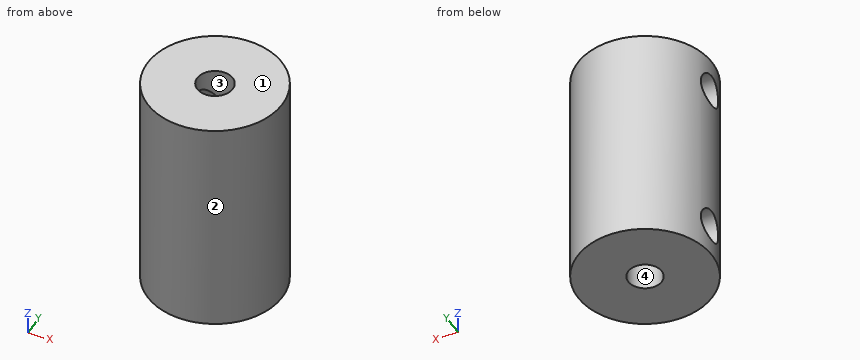
Autodesk Inventor part; units mm, degrees
ref_plane "YZ Plane" through (0, 0, 0) normal (1, 0, 0) x (0, 1, 0)
ref_plane "XZ Plane" through (0, 0, 0) normal (0, 1, 0) x (-1, 0, 0)
ref_plane "XY Plane" through (0, 0, 0) normal (0, 0, 1) x (1, 0, 0)
sketch "Sketch1" plane through (0, 0, 0) normal (0, 0, 1) x (1, 0, 0)
  circle A0 centre (0, 0) radius 6
  dimension "d0" = 12
extrude "Extrusion1" add sketch "Sketch1" along normal blind 20
sketch "Sketch2" plane through (0, 0, 20) normal (0, 0, 1) x (1, 0, 0)
  circle A0 centre (0, 0) radius 1.585
  dimension "d3" = 3.17
extrude "Extrusion2" cut sketch "Sketch2" against normal blind 10
sketch "Sketch3" plane through (0, 0, 0) normal (0, 0, -1) x (-1, 0, 0)
  circle A0 centre (0, 0) radius 1.5
  dimension "d6" = 3
extrude "Extrusion3" cut sketch "Sketch3" against normal blind 10
sketch "Sketch4" plane through (0, 0, 0) normal (1, 0, 0) x (0, 1, 0)
  circle A0 centre (0, 17) radius 1.5
  circle A1 centre (0, 3) radius 1.5
  line L0 (6, 20) -> (-6, 20)
  point P0 (0, 0)
  dimension "d9" = 3
  dimension "d10" = 3
  dimension "d11" = 3
extrude "Extrusion4" cut sketch "Sketch4" against normal through all
equation "\"d11\" = d10"
properties part number "3mm_.125inch_ShaftCoupler" material "Aluminum 6061"
Geometry check sheet. Reference: the model listing, model coordinates, mm. Face numbers are marked on the shaded views. Coordinates: 2 decimals unless noted, no trailing zeros. Write each loop counter-clockwise with the first axis right and the second up, starting at its lowest first coordinate (ties: lowest second). Pieces come first, ordered by that corner, then holes. Notation, with made-up numbers: M -29,74.5 L -25,74.5 A22 cw -25,97.5 Z; hole C -31.75,9 d6. An arc over 180 degrees is marked long. Use one line per item in the form item = value. Start each with the question number.
1) Go/stop test with a flat-tipped pin: pin 1 Ø3.5 at (x, y) = (0, 0) entering from -Z. Record where the tip stops, or that it passes through.
2) Release check for a two-part mould opening along Y. For the marked faces 1, 2, 3 and 4 record: pulls with the +Y half, pulls with the -Y half, needs draft (parallel to the pull), parting line crosses it, or undercut.
3) Section check D-D on z = 17. Enter the section's corners in (x, y) (3 decimals), and give its area (3 significant figures).
4) Section check A-A on y = 0. Enter the section's corners in (x, z) (3 decimals), and give its area (3 significant figures).
5) Thickness scan on probe 1 along X at (y, z) = (0, 12.75) (3 decimals); probe 2 along Y at (x, z) = (0, 3.5); probe 3 along X at (y, z) = (0, 16.75) (3 decimals). Record the ranges inside material, lowest first. Write a range as from..to.
6) Section check C-C on z = 5.5. Enter the section's corners in (x, y), and give its area (3 significant figures).
7) Section check B-B on x = -3.25. Enter the section's corners in (y, z).
Responses:
q1.pin_1 = 0
q2.face_1 = needs draft
q2.face_2 = parting line crosses it
q2.face_3 = undercut
q2.face_4 = undercut
q3.outline = M -5.809,-1.5 A6 ccw long -5.809,1.5 L -0.512,1.5 A1.585 cw long -0.512,-1.5 Z
q3.area = 91.3 mm2
q4.outline = M -6,0 L -1.5,0 L -1.5,1.5 L -6,1.5 Z; M -6,4.5 L -1.5,4.5 L -1.5,10 L -1.585,10 L -1.585,15.5 L -6,15.5 Z; M -6,18.5 L -1.585,18.5 L -1.585,20 L -6,20 Z; M 1.5,0 L 6,0 L 6,20 L 1.585,20 L 1.585,10 L 1.5,10 Z
q4.area = 152 mm2
q5.probe_1 = -6..-1.585, 1.585..6
q5.probe_2 = -6..-1.5, 1.5..6
q5.probe_3 = 1.585..6
q6.outline = C 0,0 d12; hole C 0,0 d3
q6.area = 106 mm2
q7.outline = M -5.04,0 L 5.04,0 L 5.04,20 L -5.04,20 Z; hole C 0,3 d3; hole C 0,17 d3
